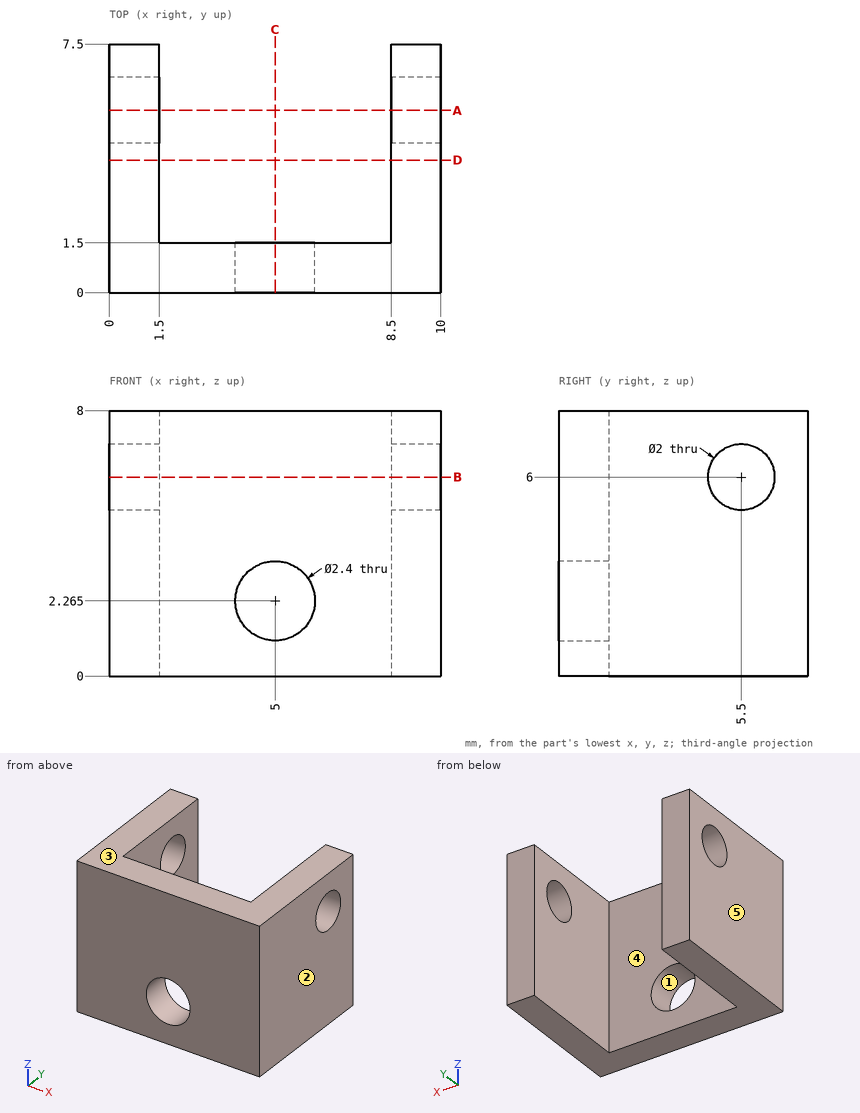
Geometry: see drawing. Coordinates: mm, zero at the bounding-box minimum. A direction names the side the tool comes from. Coordinates: 2 decimals unless noted, no trailing zeros. Order: outer loops, then holes, each group sorted by start corner. A loop starts at its lowest first (then second) coordinate and runs counter-clockwise, first axis right, second up. Notation, with made-up numbers: (12.5, -2.75) - (30.5, -2.75) arc R11 ccw to (30.5, 3.25) - close; hole circle Ø2 at (69, 20). An arc over 180 degrees is marked (long way). Return JSON: item names as keys, results as strings.
Q1. Access query for the marked faces 4 and 5. Directions: +Z, -Z, +X, -X, +Y, -Y. A direction counts if a zero-diameter tool reaches every point of the face in a straight line with its end or side. Return the directions, or none.
The answers:
{"face 4": "+Z, -Z, +Y", "face 5": "+Z, -Z, -X, +Y, -Y"}
Q2. Cut plane A-A (y = 5.5). Return loops of the section in (x, z), then the cut area to 3 significant figures.
The answers:
{"outline": "(0, 0) - (1.5, 0) - (1.5, 5) - (0, 5) - close; (0, 7) - (1.5, 7) - (1.5, 8) - (0, 8) - close; (8.5, 0) - (10, 0) - (10, 5) - (8.5, 5) - close; (8.5, 7) - (10, 7) - (10, 8) - (8.5, 8) - close", "area": "18.0 mm2"}
Q3. Draft query along Z for the marked faces 1, 2 and 3. Return one class per face: +Z half, -Z half, draft (parallel to the pull), parting line (faces both ways), or undercut.
The answers:
{"face 1": "undercut", "face 2": "draft", "face 3": "+Z half"}
Q4. Ray query, probe 1 along X at (y, z) = (2.5, 6.5); probe 2 along Y at (x, z) = (9.7, 6); probe 3 along Y at (x, z) = (8.25, 5). Return the intervals inside material, ascending.
The answers:
{"probe 1": "x = 0 to 1.5, 8.5 to 10", "probe 2": "y = 0 to 4.5, 6.5 to 7.5", "probe 3": "y = 0 to 1.5"}
Q5. Cut plane B-B (z = 6). Return loops of the section in (x, y), then the cut area to 3 significant figures.
The answers:
{"outline": "(0, 0) - (10, 0) - (10, 4.5) - (8.5, 4.5) - (8.5, 1.5) - (1.5, 1.5) - (1.5, 4.5) - (0, 4.5) - close; (0, 6.5) - (1.5, 6.5) - (1.5, 7.5) - (0, 7.5) - close; (8.5, 6.5) - (10, 6.5) - (10, 7.5) - (8.5, 7.5) - close", "area": "27.0 mm2"}
Q6. Cut plane D-D (y = 4). Return loops of the section in (x, z).
The answers:
{"outline": "(0, 0) - (1.5, 0) - (1.5, 8) - (0, 8) - close; (8.5, 0) - (10, 0) - (10, 8) - (8.5, 8) - close"}
Q7. Cut plane C-C (x = 5). Return loops of the section in (y, z) (1 decimal).
The answers:
{"outline": "(0, 0) - (1.5, 0) - (1.5, 1.1) - (0, 1.1) - close; (0, 3.5) - (1.5, 3.5) - (1.5, 8) - (0, 8) - close"}
